Verification items for this drawing (mm, ordinates from the low corner). Coordinates: 2 decimals unless noted, no trailing zeros. Loops run counter-clockwise (first coordinate to the right, second up) from the corner with the lowest first, then second, coordinate; pieces in that order, holes last. Notation, with made-up numbers: M 2,45 L 50,45 A14 cw 50,63 Z; hole C 76.5,88 d5. An arc over 180 degrees is marked long. Return JSON: item names as keys, results as strings.
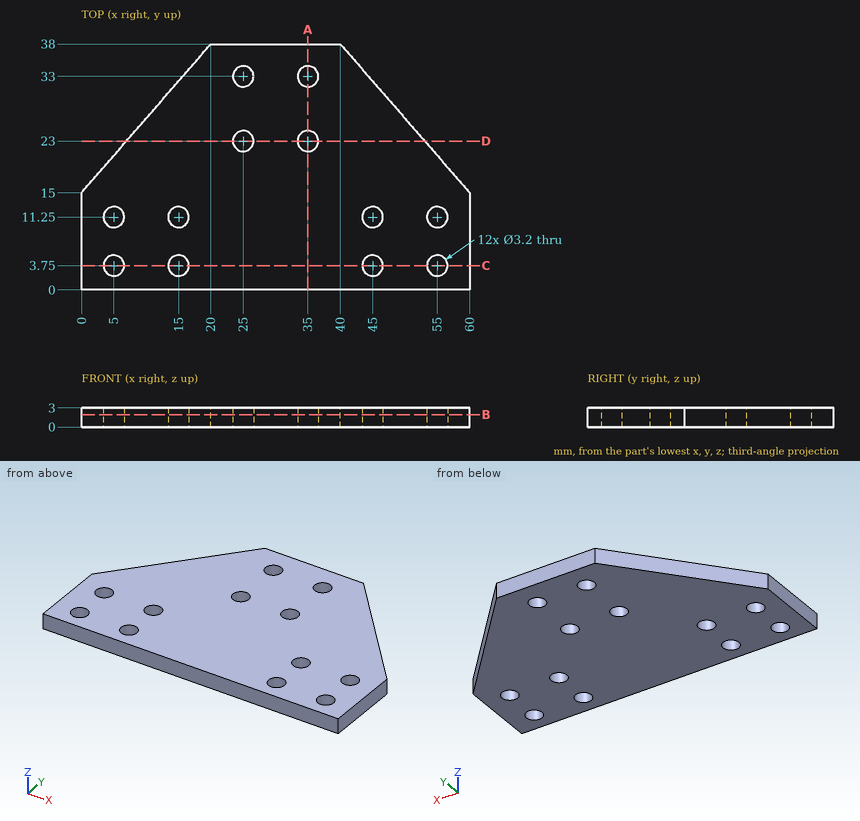
1) Go/stop test with a flat-tipped pin: pin 1 Ø2.5 at (x, y) = (45, 3.75) entering from +Z. Record where the tip stops, or that it passes through.
Answers:
{"pin 1": "through"}
2) Section check B-B on z = 1.95. Count the separate pieces of the cut face and the enclosed holes in it, then the cut area to 3 significant figures.
Answers:
{"separate pieces": "1", "enclosed holes": "12", "area": "1,720 mm²"}
3) Section check C-C on y = 3.75. Record the cut outline in (x, z).
Answers:
{"outline": "M 0,0 L 3.4,0 L 3.4,3 L 0,3 Z; M 6.6,0 L 13.4,0 L 13.4,3 L 6.6,3 Z; M 16.6,0 L 43.4,0 L 43.4,3 L 16.6,3 Z; M 46.6,0 L 53.4,0 L 53.4,3 L 46.6,3 Z; M 56.6,0 L 60,0 L 60,3 L 56.6,3 Z"}
4) Scan lines: line 1 along Y through (x, z) = (25, 0.75); line 2 along Y through (x, z) = (45, 1.9); line 3 along X through (y, z) = (22, 1.2). Record each from-to range of solid material in increasing order. Write a range as [from, to].
Answers:
{"line 1": "[0, 21.4], [24.6, 31.4], [34.6, 38]", "line 2": "[0, 2.15], [5.35, 9.65], [12.85, 32.25]", "line 3": "[6.09, 23.75], [26.25, 33.75], [36.25, 53.91]"}
5) Section check D-D on y = 23. Record the cut outline in (x, z), then the cut area to 3 significant figures.
Answers:
{"outline": "M 6.96,0 L 23.4,0 L 23.4,3 L 6.96,3 Z; M 26.6,0 L 33.4,0 L 33.4,3 L 26.6,3 Z; M 36.6,0 L 53.04,0 L 53.04,3 L 36.6,3 Z", "area": "119 mm²"}
6) Section check A-A on x = 35. Record the cut outline in (y, z).
Answers:
{"outline": "M 0,0 L 21.4,0 L 21.4,3 L 0,3 Z; M 24.6,0 L 31.4,0 L 31.4,3 L 24.6,3 Z; M 34.6,0 L 38,0 L 38,3 L 34.6,3 Z"}
